Could you check a few things on this model? Use its own coordinates, in mm. Face numbers are marked on the shaded views. Give positions to 0.01 mm unless a question says otherwise; leave off trailing zeros. Order: outer loops, then holes, each group sorted by start corner. A loop starts at its lowest first (then second) coordinate and runs counter-clockwise, first axis right, second up. Notation, with made-up numbers: (-21.5, 0) - (26.5, 0) arc R22 cw to (26.5, 23) - close; hole circle Ø4 at (-13, 73.25). An arc over 180 degrees is marked (long way). One line per question, with ' | ' between items. Start each with the question number.
1. Imagine slicing it at A-A (z = 330.2). Give the number of separate pieces and of enclosed holes in the cut face, and give its area (3 significant figures).
2. If we mould it in two halves opening along X, with no side actions, what happens to the marked faces 1 and 2? For each: released by +X, released by -X, zero draft, split by the parting line, or undercut.
3. I need wall thicknesses on probe 1 along Z at (x, y) = (-444.5, -1.75); probe 2 along Z at (x, y) = (-330.2, -3.75); probe 3 along Z at (x, y) = (-347, -3.5). Which ranges of each line are inside material? Lowest first, please. Write a range as from..to.
4. Imagine slicing it at C-C (z = 197). Please give me the cut outline in (x, y), and give its area (3 significant figures).
5. For P1, Ø2.5, axis at x = -408.5, y = 6.5, coming from the +Z side; P2, Ø5, axis at x = -285.5, y = 4, coming from the +Z side, each with a flat end and sliding along its axis, tell me the tip position at first contact or that it passes through.
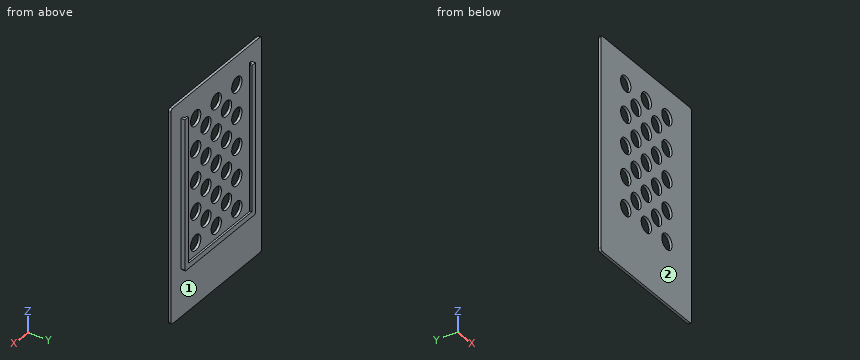
```python
from build123d import *

# Parameters (mm, degrees)
F1_DEPTH = 9.525
F2_DEPTH = 4.7625
F3_DEPTH = 9.525
F0_W     = 234.95
F0_H     = 358.3939369202
F0_R     = 19.05
F4_DEPTH = 6.35


with BuildPart() as f1:
    # F0 (on Front) → F1 (new body)
    with BuildSketch(Plane.XZ):
        Polygon((-524.0142820795, 625.0939369202), (-530.3642820795, 625.0939369202), (-530.3642820795, 260.35), (-282.7142820795, 260.35), (-282.7142820795, 625.0939369202), (-289.0642820795, 625.0939369202), (-289.0642820795, 266.7), (-524.0142820795, 266.7), align=None)
    extrude(amount=-F1_DEPTH)

    # F0 (on Front) → F2 (cut)
    with BuildSketch(Plane.XZ):
        Polygon((-524.0142820795, 625.0939369202), (-530.3642820795, 625.0939369202), (-530.3642820795, 260.35), (-282.7142820795, 260.35), (-282.7142820795, 625.0939369202), (-289.0642820795, 625.0939369202), (-289.0642820795, 266.7), (-524.0142820795, 266.7), align=None)
    extrude(amount=-F2_DEPTH, mode=Mode.SUBTRACT)

    # F0 (on Front) → F3 (join)
    with BuildSketch(Plane.XZ):
        with BuildLine():
            ThreePointArc((-536.7142820795, 257.175), (-535.7843461097, 254.9299359697), (-533.5392820795, 254))
            Line((-533.5392820795, 254), (-279.5392820795, 254))
            ThreePointArc((-279.5392820795, 254), (-277.2942180492, 254.9299359697), (-276.3642820795, 257.175))
            Line((-276.3642820795, 257.175), (-276.3642820795, 625.0939369202))
            Line((-276.3642820795, 625.0939369202), (-282.7142820795, 625.0939369202))
            Line((-282.7142820795, 625.0939369202), (-282.7142820795, 260.35))
            Line((-282.7142820795, 260.35), (-530.3642820795, 260.35))
            Line((-530.3642820795, 260.35), (-530.3642820795, 625.0939369202))
            Line((-530.3642820795, 625.0939369202), (-536.7142820795, 625.0939369202))
            Line((-536.7142820795, 625.0939369202), (-536.7142820795, 257.175))
        make_face()
    extrude(amount=-F3_DEPTH)

    # F0 (on Front) → F4 (join)
    with BuildSketch(Plane.XZ):
        with BuildLine():
            ThreePointArc((-568.4642820795, 666.75), (-572.95441014, 664.8901280605), (-574.8142820795, 660.4))
            Line((-574.8142820795, 660.4), (-574.8142820795, 146.05))
            ThreePointArc((-574.8142820795, 146.05), (-572.95441014, 141.5598719395), (-568.4642820795, 139.7))
            Line((-568.4642820795, 139.7), (-244.6142820795, 139.7))
            ThreePointArc((-244.6142820795, 139.7), (-240.1241540189, 141.5598719395), (-238.2642820795, 146.05))
            Line((-238.2642820795, 146.05), (-238.2642820795, 660.4))
            ThreePointArc((-238.2642820795, 660.4), (-240.1241540189, 664.8901280605), (-244.6142820795, 666.75))
            Line((-244.6142820795, 666.75), (-568.4642820795, 666.75))
        make_face()
        with BuildLine():
            Line((-279.5392820795, 254), (-533.5392820795, 254))
            ThreePointArc((-533.5392820795, 254), (-535.7843461097, 254.9299359697), (-536.7142820795, 257.175))
            Line((-536.7142820795, 257.175), (-536.7142820795, 625.0939369202))
            Line((-536.7142820795, 625.0939369202), (-530.3642820795, 625.0939369202))
            Line((-530.3642820795, 625.0939369202), (-524.0142820795, 625.0939369202))
            Line((-524.0142820795, 625.0939369202), (-289.0642820795, 625.0939369202))
            Line((-289.0642820795, 625.0939369202), (-282.7142820795, 625.0939369202))
            Line((-282.7142820795, 625.0939369202), (-276.3642820795, 625.0939369202))
            Line((-276.3642820795, 625.0939369202), (-276.3642820795, 257.175))
            ThreePointArc((-276.3642820795, 257.175), (-277.2942180492, 254.9299359697), (-279.5392820795, 254))
        make_face(mode=Mode.SUBTRACT)
        with Locations((-406.5392820795, 445.8969684601)):
            Rectangle(F0_W, F0_H)
        with Locations((-482.6, 292.1)):
            Circle(F0_R, mode=Mode.SUBTRACT)
        with Locations((-444.5, 330.2)):
            Circle(F0_R, mode=Mode.SUBTRACT)
        with Locations((-482.6, 368.3)):
            Circle(F0_R, mode=Mode.SUBTRACT)
        with Locations((-406.4, 292.1)):
            Circle(F0_R, mode=Mode.SUBTRACT)
        with Locations((-368.3, 330.2)):
            Circle(F0_R, mode=Mode.SUBTRACT)
        with Locations((-330.2, 292.1)):
            Circle(F0_R, mode=Mode.SUBTRACT)
        with Locations((-406.4, 368.3)):
            Circle(F0_R, mode=Mode.SUBTRACT)
        with Locations((-330.2, 368.3)):
            Circle(F0_R, mode=Mode.SUBTRACT)
        with Locations((-482.6, 444.5)):
            Circle(F0_R, mode=Mode.SUBTRACT)
        with Locations((-444.5, 406.4)):
            Circle(F0_R, mode=Mode.SUBTRACT)
        with Locations((-482.6, 520.7)):
            Circle(F0_R, mode=Mode.SUBTRACT)
        with Locations((-444.5, 482.6)):
            Circle(F0_R, mode=Mode.SUBTRACT)
        with Locations((-482.6, 596.9)):
            Circle(F0_R, mode=Mode.SUBTRACT)
        with Locations((-444.5, 558.8)):
            Circle(F0_R, mode=Mode.SUBTRACT)
        with Locations((-368.3, 406.4)):
            Circle(F0_R, mode=Mode.SUBTRACT)
        with Locations((-406.4, 444.5)):
            Circle(F0_R, mode=Mode.SUBTRACT)
        with Locations((-330.2, 444.5)):
            Circle(F0_R, mode=Mode.SUBTRACT)
        with Locations((-368.3, 482.6)):
            Circle(F0_R, mode=Mode.SUBTRACT)
        with Locations((-406.4, 520.7)):
            Circle(F0_R, mode=Mode.SUBTRACT)
        with Locations((-330.2, 520.7)):
            Circle(F0_R, mode=Mode.SUBTRACT)
        with Locations((-368.3, 558.8)):
            Circle(F0_R, mode=Mode.SUBTRACT)
        with Locations((-406.4, 596.9)):
            Circle(F0_R, mode=Mode.SUBTRACT)
        with Locations((-330.2, 596.9)):
            Circle(F0_R, mode=Mode.SUBTRACT)
        Polygon((-524.0142820795, 625.0939369202), (-530.3642820795, 625.0939369202), (-530.3642820795, 260.35), (-282.7142820795, 260.35), (-282.7142820795, 625.0939369202), (-289.0642820795, 625.0939369202), (-289.0642820795, 266.7), (-524.0142820795, 266.7), align=None)
        with BuildLine():
            ThreePointArc((-536.7142820795, 257.175), (-535.7843461097, 254.9299359697), (-533.5392820795, 254))
            Line((-533.5392820795, 254), (-279.5392820795, 254))
            ThreePointArc((-279.5392820795, 254), (-277.2942180492, 254.9299359697), (-276.3642820795, 257.175))
            Line((-276.3642820795, 257.175), (-276.3642820795, 625.0939369202))
            Line((-276.3642820795, 625.0939369202), (-282.7142820795, 625.0939369202))
            Line((-282.7142820795, 625.0939369202), (-282.7142820795, 260.35))
            Line((-282.7142820795, 260.35), (-530.3642820795, 260.35))
            Line((-530.3642820795, 260.35), (-530.3642820795, 625.0939369202))
            Line((-530.3642820795, 625.0939369202), (-536.7142820795, 625.0939369202))
            Line((-536.7142820795, 625.0939369202), (-536.7142820795, 257.175))
        make_face()
    extrude(amount=F4_DEPTH)


solid = f1.part
```
Results found:
1) separate pieces: 3 | enclosed holes: 0 | area: 1,830 mm2
2) face 1: undercut | face 2: zero draft
3) probe 1: z = 139.7..311.15, 349.25..387.35, 425.45..463.55, 501.65..539.75, 577.85..666.75 | probe 2: z = 139.7..273.05, 311.15..349.25, 387.35..425.45, 463.55..501.65, 539.75..577.85, 615.95..666.75 | probe 3: z = 139.7..283.12, 301.08..359.32, 377.28..435.52, 453.48..511.72, 529.68..587.92, 605.88..666.75
4) outline: (-574.81, -6.35) - (-238.26, -6.35) - (-238.26, 0) - (-574.81, 0) - close | area: 2,140 mm2
5) P1: stops at z = 266.7 | P2: stops at z = 625.09
